Autodesk Inventor part; units mm, degrees
ref_plane "YZ Plane" through (0, 0, 0) normal (1, 0, 0) x (0, 1, 0)
ref_plane "XZ Plane" through (0, 0, 0) normal (0, 1, 0) x (-1, 0, 0)
ref_plane "XY Plane" through (0, 0, 0) normal (0, 0, 1) x (1, 0, 0)
sketch "Skizze1" plane through (0, 0, 0) normal (0, 1, 0) x (-1, 0, 0)
  line L0 (15.1, 14.35) -> (-15.1, 14.35)
  line L1 (-15.1, 14.35) -> (-15.1, 2.05)
  line L2 (-15.1, 2.05) -> (15.1, 2.05)
  line L3 (15.1, 2.05) -> (15.1, 14.35)
  line L4 (15.1, 14.35) -> (-15.1, 2.05) construction
  line L5 (-15.1, 14.35) -> (15.1, 2.05) construction
  line L6 (15.1, -2.05) -> (-15.1, -2.05)
  line L7 (-15.1, -2.05) -> (-15.1, -14.35)
  line L8 (-15.1, -14.35) -> (15.1, -14.35)
  line L9 (15.1, -14.35) -> (15.1, -2.05)
  line L10 (15.1, -2.05) -> (-15.1, -14.35) construction
  line L11 (-15.1, -2.05) -> (15.1, -14.35) construction
  line L12 (28.45, 18) -> (-28.45, 18)
  line L13 (-28.45, 18) -> (-28.45, -18)
  line L14 (-28.45, -18) -> (28.45, -18)
  line L15 (28.45, -18) -> (28.45, 18)
  line L16 (28.45, 18) -> (-28.45, -18) construction
  line L17 (-28.45, 18) -> (28.45, -18) construction
  point P0 (0, 0)
  point P1 (0, 8.2)
  point P2 (0, -8.2)
  dimension "d0" = 30.2
  dimension "d1" = 12.3
  dimension "d2" = 30.2
  dimension "d3" = 12.3
  dimension "d5" = 4.1
  dimension "d6" = 2.05
  dimension "d7" = 56.9
  dimension "d8" = 36
extrude "Extrusion1" add sketch "Skizze1" along normal blind 3
chamfer "Fase1" distance 2 angle 45 4 edges at (0, 0, 2.05) (0, 0, -14.35) (0, 0, -2.05) (0, 0, 14.35)
sketch "Skizze2" plane through (0, 3, 0) normal (0, 1, 0) x (1, 0, 0)
  line L0 (28.45, 18) -> (-28.45, 18)
  line L1 (-25.65, -18) -> (25.65, -18)
  line L2 (25.65, -18) -> (25.65, 18)
  line L3 (25.65, 18) -> (-25.65, 18)
  line L4 (-25.65, 18) -> (-25.65, -18)
  line L5 (-25.65, -18) -> (25.65, 18) construction
  line L6 (25.65, -18) -> (-25.65, 18) construction
  line L7 (-25.65, 0) -> (25.65, 0)
  point P0 (0, 0)
  dimension "d14" = 51.3
hole "Bohrung1" at (-25.65, 3, 0) at (25.65, 3, 0) direction (0, -1, 0) diameter 2.4 end through all countersink diameter 4.4 countersink angle 90
fillet "Rundung1" radius 13 4 edges at (28.45, 1.5, -18) (28.45, 1.5, 18) (-28.45, 1.5, -18) (-28.45, 1.5, 18)
properties part number "Wago2Din_2Way"
Model file for the job. Use its own axes, mm. A direction names the side the tool comes from. Round coordinates to 2 decimals unless told otherwise and drop trailing zeros. Order: outer loops, then holes, each group sorted by start corner. A loop starts at its lowest first (then second) coordinate and runs counter-clockwise, first axis right, second up. Notation, with made-up numbers: M -29.5,-20.5 L -5.5,-20.5 A18 cw -5.5,-2.5 Z; hole C 65.25,35 d10. An arc over 180 degrees is marked long. Use CSV: the item, a comma, the result in double quotes.
Item 1: Saw through at D-D (x = 25.65). List the corners of the cut face in (y, z), plus the area to 3 significant figures.
Worked answers:
outline,"M 0,-13.06 L 3,-13.06 L 3,-2.2 L 2,-1.2 L 0,-1.2 Z; M 0,1.2 L 2,1.2 L 3,2.2 L 3,13.06 L 0,13.06 Z"
area,"70.2 mm²"
Item 2: Pin check, flat tips, straight feed: pin 1 (1.5 mm diameter, centred on y = 2, z = 13, fed in from -X); pin 2 (4 mm diameter, centred on x = -5.5, z = -4, fed in from -Y); pin 3 (1.5 mm diameter, centred on y = 2, z = 12, fed in from -X). Stop position of each tip, or through.
Worked answers:
pin 1,"x = -26.24"
pin 2,"y = 1.95"
pin 3,"x = -26.85"
Item 3: Saw through at B-B (z = -4). List the corners of the cut face in (x, y), plus the area to 3 significant figures.
Worked answers:
outline,"M -28.45,0 L -15.1,0 L -15.1,3 L -28.45,3 Z; M 15.1,0 L 28.45,0 L 28.45,3 L 15.1,3 Z"
area,"80.1 mm²"
Item 4: Saw through at C-C (y = 0.6). List the corners of the cut face in (x, z), plus the area to 3 significant figures.
Worked answers:
outline,"M -28.45,-5 A13 ccw -15.45,-18 L 15.45,-18 A13 ccw 28.45,-5 L 28.45,5 A13 ccw 15.45,18 L -15.45,18 A13 ccw -28.45,5 Z; hole C -25.65,0 d2.4; hole M -15.1,-15.75 L 15.1,-15.75 L 15.1,-0.65 L -15.1,-0.65 Z; hole M -15.1,0.65 L 15.1,0.65 L 15.1,15.75 L -15.1,15.75 Z; hole C 25.65,0 d2.4"
area,"982 mm²"
Item 5: Saw through at A-A (x = 3.5). List the corners of the cut face in (y, z), plus the area to 3 significant figures.
Worked answers:
outline,"M 0,-18 L 3,-18 L 3,-14.35 L 2,-14.35 L 0,-16.35 Z; M 0,-0.05 L 2,-2.05 L 3,-2.05 L 3,2.05 L 2,2.05 L 0,0.05 Z; M 0,16.35 L 2,14.35 L 3,14.35 L 3,18 L 0,18 Z"
area,"26.2 mm²"
Item 6: Probe probe 1 along X at (y, z) = (0.4, 0); probe 2 along Z at (x, y) = (11.5, 2.7); probe 3 along Z at (x, y) = (4.5, 0.45). List the from-to ranges inside material, lowest first.
Worked answers:
probe 1,"-28.45 to -26.85, -24.45 to 24.45, 26.85 to 28.45"
probe 2,"-18 to -14.35, -2.05 to 2.05, 14.35 to 18"
probe 3,"-18 to -15.9, -0.5 to 0.5, 15.9 to 18"
Item 7: Pull direction Z, two halves, no side cores. Call faces 3 (the face through (-19, 0, 0)), 4 (the face through (0, 1, 18)), 5 (the face through (-0.21, 0.99, 1.04)): released by +Z, released by -Z, zero draft, split by the parting line, or undercut.
Worked answers:
face 3,"zero draft"
face 4,"released by +Z"
face 5,"undercut"
Item 8: Which spindle directions (+Z, -Z, +X, -X, +Y, -Y) get a long thin tool onto all of the face, cutting with end or side? Do faces 1 (the face through (-0.21, 0.99, -15.36)), 2 (the face through (24.46, 0.99, -0.16)). Say none if no direction does.
Worked answers:
face 1,"-Y"
face 2,"+Y, -Y"
